Part model, mm, in its own coordinate system. A direction names the side the tool comes from. Round coordinates to 2 decimals unless told otherwise and drop trailing zeros. Write each loop counter-clockwise with the first axis right and the second up, starting at its lowest first coordinate (ties: lowest second). Pieces come first, ordered by that corner, then holes.
1) Pull direction Y, two halves, no side cores. Call faces 5 (the flat face through (0, 86, -197)), 6 (the flat face through (150, 0, -203)), 7 (the flat face through (20, 173, -215)): +Y half, -Y half, draft (parallel to the pull), parting line (faces both ways), or undercut.
2) Drill centre lines: L1, parallel to X at y = 32.5, z = -162; L2, parallel to Z at x = 107.5, y = 149; L3, parallel to Y at x = 119.5, z = -382. Where is each one in solid material? Low to high.
3) Saw through at A-A on y = 110.5. Write the cut outline in (x, z).
4) Saw through at B-B on z = -234.5. Write the cut outline in (x, y), and give its area (3 significant figures).
5) Which spindle directions (+Z, -Z, +X, -X, +Y, -Y) get a long thin tool onto all of the face, cutting with end or side? Do faces 1 (the flat face through (280, 184, -198)), 2 (the flat face through (151, 186, -377)), 3 (the flat face through (151, 186, -23)), 4 (the flat face through (150, 86, -2)). Say none if no direction does.
6) Flat gauge pins, fed straight in: pin 1 (5.5 mm diameter, centred on y = 181.5, z = -257, fed in from +X); pin 2 (20 mm diameter, centred on x = 176.5, y = 187, fed in from +Z); pin 3 (11 mm diameter, centred on x = 136.5, y = 189, fed in from -Z). Where does each tip first touch, or does it go through?
7) Saw through at C-C on x = 79. Write the cut outline in (y, z), and give its area (3 significant figures).
```python
from build123d import *

# Parameters (mm, degrees)
SKETCH1_W           = 305
SKETCH1_H           = 400
BOSS_EXTRUDE1_DEPTH = 175
SHELL1_T            = 2
SKETCH2_W           = 255
SKETCH2_H           = 350
CUT_EXTRUDE1_DEPTH  = 5
SKETCH3_W           = 259
SKETCH3_H           = 354
SKETCH3_W_2         = 255
SKETCH3_H_2         = 350
BOSS_EXTRUDE2_DEPTH = 20
FILLET1_R           = 2


with BuildPart() as part:
    # Sketch1 → Boss-Extrude1 (new body)
    with BuildSketch(Plane(origin=(0, 0, 0), x_dir=(1, 0, 0), z_dir=(0, 1, 0))):
        with Locations((152.5, 200)):
            Rectangle(SKETCH1_W, SKETCH1_H)
    extrude(amount=BOSS_EXTRUDE1_DEPTH)

    # Shell1 (no face opened: a closed hollow body)
    add(offset(amount=-SHELL1_T, mode=Mode.PRIVATE), mode=Mode.SUBTRACT)

    # Sketch2 → Cut-Extrude1 (cut)
    with BuildSketch(Plane(origin=(0, 175, 0), x_dir=(1, 0, 0), z_dir=(0, 1, 0))):
        with Locations((152.5, 200)):
            Rectangle(SKETCH2_W, SKETCH2_H)
    extrude(amount=-CUT_EXTRUDE1_DEPTH, mode=Mode.SUBTRACT)

    # Sketch3 → Boss-Extrude2 (add)
    with BuildSketch(Plane(origin=(0, 175, 0), x_dir=(1, 0, 0), z_dir=(0, 1, 0))):
        with Locations((152.5, 200)):
            Rectangle(SKETCH3_W, SKETCH3_H)
        with Locations((152.5, 200)):
            Rectangle(SKETCH3_W_2, SKETCH3_H_2, mode=Mode.SUBTRACT)
    extrude(amount=BOSS_EXTRUDE2_DEPTH)

    # Fillet1
    fillet1_edges = [part.edges().sort_by_distance(p)[0] for p in [
        (305, 175, -200),
        (2, 2, -200),
        (2, 87.5, -398),
        (152.5, 2, -2),
        (2, 87.5, -2),
        (303, 2, -200),
        (303, 87.5, -2),
        (152.5, 2, -398),
        (303, 87.5, -398),
        (2, 173, -200),
        (152.5, 173, -2),
        (303, 173, -200),
        (152.5, 173, -398),
        (152.5, 175, -400),
        (23, 175, -200),
        (0, 175, -200),
        (152.5, 0, -400),
        (23, 185, -377),
        (152.5, 175, -23),
        (23, 185, -23),
        (282, 175, -200),
        (282, 185, -23),
        (152.5, 175, -377),
        (282, 185, -377),
        (305, 0, -200),
        (152.5, 0, 0),
        (0, 0, -200),
        (0, 87.5, -400),
        (305, 87.5, -400),
        (305, 87.5, 0),
        (0, 87.5, 0),
        (152.5, 175, 0),
    ]]
    fillet(fillet1_edges, radius=FILLET1_R)


solid = part.part
```
Completed:
1. face 5: draft
1. face 6: -Y half
1. face 7: undercut
2. L1: x = 0 to 2, 303 to 305
2. L2: z = -400 to -398, -2 to 0
2. L3: y = 0 to 2, 173 to 175
3. outline: (0, -398) arc R2 ccw to (2, -400) - (303, -400) arc R2 ccw to (305, -398) - (305, -2) arc R2 ccw to (303, 0) - (2, 0) arc R2 ccw to (0, -2) - close; hole (2, -396) arc R2 ccw to (4, -398) - (301, -398) arc R2 ccw to (303, -396) - (303, -4) arc R2 ccw to (301, -2) - (4, -2) arc R2 ccw to (2, -4) - close
4. outline: (0, 2) arc R2 ccw to (2, 0) - (303, 0) arc R2 ccw to (305, 2) - (305, 173) arc R2 ccw to (303, 175) - (284, 175) arc R2 cw to (282, 177) - (282, 195) - (280, 195) - (280, 173) - (301, 173) arc R2 cw to (303, 171) - (303, 4) arc R2 cw to (301, 2) - (4, 2) arc R2 cw to (2, 4) - (2, 171) arc R2 cw to (4, 173) - (25, 173) - (25, 195) - (23, 195) - (23, 177) arc R2 cw to (21, 175) - (2, 175) arc R2 ccw to (0, 173) - close
4. area: 1,480 mm2
5. face 1: +Y
5. face 2: -Z, +X, -X, +Y
5. face 3: +Z, +X, -X, +Y
5. face 4: none
6. pin 1: stops at x = 282
6. pin 2: stops at z = -23
6. pin 3: stops at z = -377
7. outline: (0, -398) arc R2 ccw to (2, -400) - (173, -400) arc R2 ccw to (175, -398) - (175, -379) arc R2 cw to (177, -377) - (195, -377) - (195, -375) - (173, -375) - (173, -396) arc R2 cw to (171, -398) - (4, -398) arc R2 cw to (2, -396) - (2, -4) arc R2 cw to (4, -2) - (171, -2) arc R2 cw to (173, -4) - (173, -25) - (195, -25) - (195, -23) - (177, -23) arc R2 cw to (175, -21) - (175, -2) arc R2 ccw to (173, 0) - (2, 0) arc R2 ccw to (0, -2) - close
7. area: 1,670 mm2
